Part print with two shaded views. Sizes in mm from the minimum x, y, z corner. Give positions to 0.01 mm unless a question says otherwise; leave off trailing zeros. Order: outer loops, then holes, each group sorted by start corner. A loop starts at its lowest first (then second) coordinate and runs counter-clockwise, first axis right, second up. Notation, with made-up numbers: M 47,78 L 53,78 A8 cw 53,88 Z; hole C 47.5,-12 d6. An arc over 180 degrees is marked long. Answer as CSV lines item,"result".
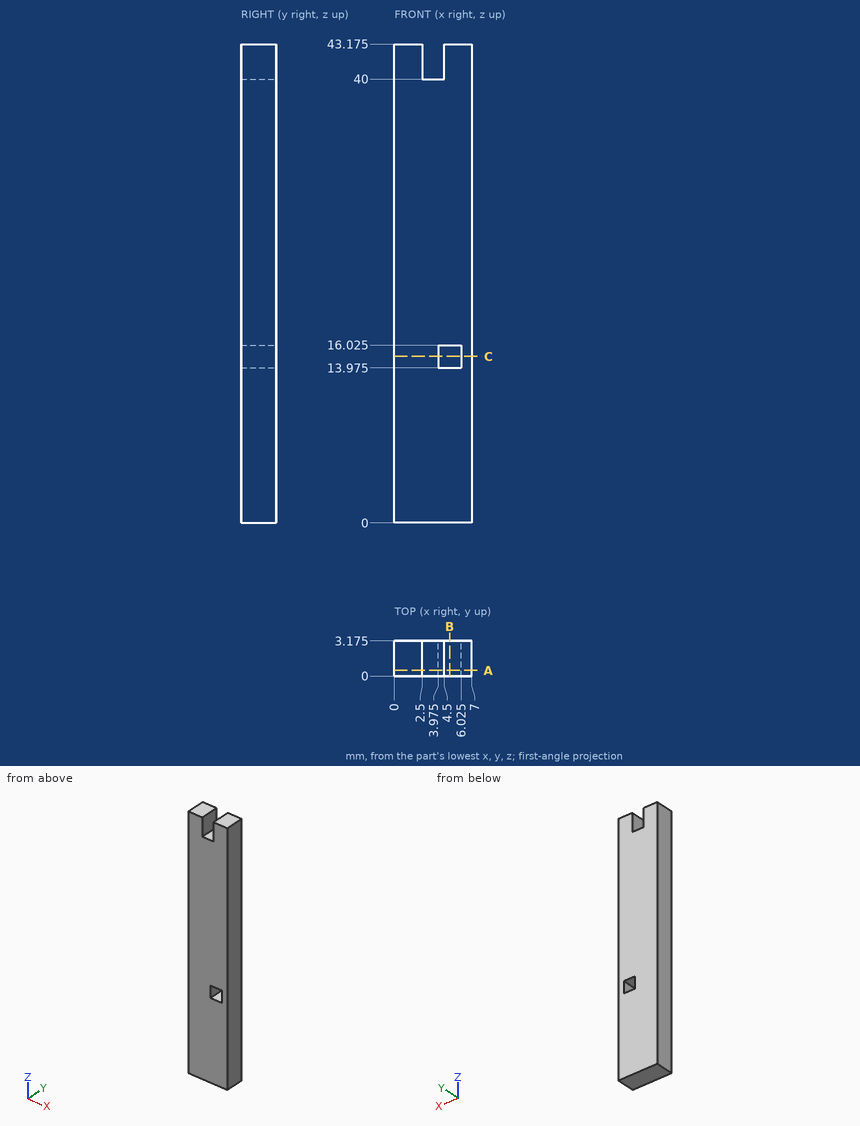
Item 1: Band-saw the part on B-B (x = 5). Give the cut face in (y, z) (3 decimals), and give its area (3 significant figures).
Geometry says:
outline,"M 0,0 L 3.175,0 L 3.175,13.975 L 0,13.975 Z; M 0,16.025 L 3.175,16.025 L 3.175,43.175 L 0,43.175 Z"
area,"131 mm2"
Item 2: Probe line 1 along Z through (x, y) = (5.75, 1.55) (3 decimals); line 2 along Z through (x, y) = (4.25, 1.8) (3 decimals); line 3 along Z through (x, y) = (2.75, 2.6). List the from-to ranges inside material, lowest first. Write a range as from..to.
Geometry says:
line 1,"z = 0..13.975, 16.025..43.175"
line 2,"z = 0..13.975, 16.025..40"
line 3,"z = 0..40"
Item 3: Band-saw the part on C-C (z = 15). Give the cut face in (x, y) (3 decimals), and give its area (3 significant figures).
Geometry says:
outline,"M 0,0 L 3.975,0 L 3.975,3.175 L 0,3.175 Z; M 6.025,0 L 7,0 L 7,3.175 L 6.025,3.175 Z"
area,"15.7 mm2"
Item 4: Band-saw the part on A-A (y = 0.5). Give the cut face in (x, z) (3 decimals), and give its area (3 significant figures).
Geometry says:
outline,"M 0,0 L 7,0 L 7,43.175 L 4.5,43.175 L 4.5,40 L 2.5,40 L 2.5,43.175 L 0,43.175 Z; hole M 3.975,13.975 L 6.025,13.975 L 6.025,16.025 L 3.975,16.025 Z"
area,"292 mm2"
Item 5: Drop a flat-ended pin along its axis: pin 1 (1.5 mm diameter, centred on y = 1.5, z = 33, fed in from -X). Give the stop position or say it passes through.
Geometry says:
pin 1,"stops at x = 0"
